Input: part model. Units: mm. Frame: model coordinates. Give positions to 0.01 mm unless a question says otherwise; leave off trailing zeros. Loops run counter-clockwise (first coordinate to the right, second up) from the corner with the lowest first, then second, coordinate; pieces in that order, holes last. Notation, with made-up numbers: (35, 75.25) -> (46, 75.25) arc R10 cw to (46, 94.25) -> close; hole circle Ø3 at (-37.75, 8.5). An arc over 180 degrees is marked (long way). Answer as a JSON object with one key per item and string values. Group by question number.
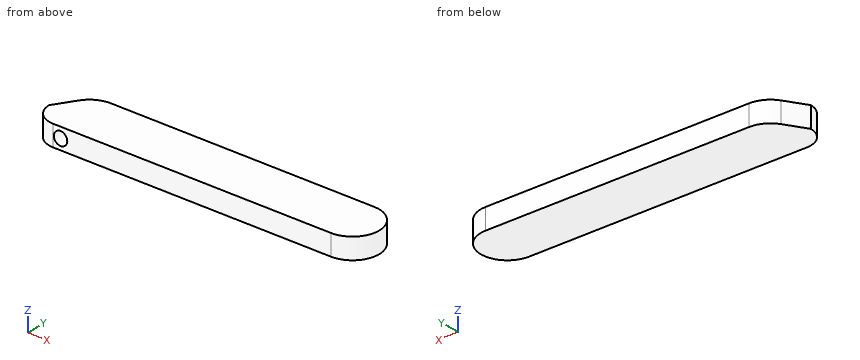
```python
from build123d import *

# Parameters (mm, degrees)
BOSS_EXTRUDE1_DEPTH = 8
SKETCH4_R           = 2.55
CUT_EXTRUDE1_DEPTH  = 7


with BuildPart() as part:
    # Sketch2 → Boss-Extrude1 (new body)
    with BuildSketch(Plane.XY):
        with BuildLine():
            Line((-50.683757693, 15.376803881), (49.316242307, 15.376803881))
            ThreePointArc((49.316242307, 15.376803881), (59.496208487, 5.196837701), (49.316242307, -4.98312848))
            Line((49.316242307, -4.98312848), (-56.12878489, -4.98312848))
            ThreePointArc((-56.12878489, -4.98312848), (-61.779081531, -2.642698979), (-64.119511032, 3.007597662))
            Line((-64.119511032, 3.007597662), (-59.08344563, 10.803150955))
            ThreePointArc((-59.08344563, 10.803150955), (-55.465835132, 14.15927138), (-50.683757693, 15.376803881))
        make_face()
    extrude(amount=BOSS_EXTRUDE1_DEPTH)

    # Sketch4 → Cut-Extrude1 (cut)
    with BuildSketch(Plane.XZ.offset(4.98312848)):
        with Locations((-53.279822917, 4)):
            Circle(SKETCH4_R)
    extrude(amount=-CUT_EXTRUDE1_DEPTH, mode=Mode.SUBTRACT)


solid = part.part
```
Q1. Ray query, probe 1 along X at (y, z) = (1, 5.5); probe 2 along X at (y, z) = (1.75, 3.75); probe 3 along Y at (x, z) = (50, 7.5). Return the intervals inside material, ascending.
Q2. Section C-C on y = 9.75. Return the cut outline in (x, z).
Q3. Pin query (flat end, axial travel): pin 1 Ø4 at (y, z) = (8.5, 1.5) entering from +X; pin 2 Ø2 at (y, z) = (12.5, 6) entering from -X. Return the tip coordinate at first contact, or that it passes through.
Q4. Section A-A on z = 4. Return the cut outline in (x, y).
Q5. Section B-B on y = -2. Return the cut outline in (x, z), then the cut area to 3 significant figures.
Numbers:
{
 "1": {"probe 1": "x = -63.86 to -55.34, -51.22 to 58.59", "probe 2": "x = -64.02 to -55.82, -50.74 to 58.89", "probe 3": "y = -4.96 to 15.35"},
 "2": {"outline": "(-59.76, 0) -> (58.42, 0) -> (58.42, 8) -> (-59.76, 8) -> close"},
 "3": {"pin 1": "stops at x = 59.41", "pin 2": "stops at x = -58.59"},
 "4": {"outline": "(-64.12, 3.01) arc R7.99 ccw to (-56.13, -4.98) -> (-55.83, -4.98) -> (-55.83, 2.02) -> (-50.73, 2.02) -> (-50.73, -4.98) -> (49.32, -4.98) arc R10.18 ccw to (49.32, 15.38) -> (-50.68, 15.38) arc R10 ccw to (-59.08, 10.8) -> close"},
 "5": {"outline": "(-62.36, 0) -> (56.52, 0) -> (56.52, 8) -> (-62.36, 8) -> close; hole circle Ø5.1 at (-53.28, 4)", "area": "931 mm²"}
}
